Print and shaded views of the part. All mm, measured from the part's lowest x, y and z. A direction names the side the tool comes from. Round coordinates to 2 decimals unless told otherwise and drop trailing zeros. Write each loop counter-clockwise with the first axis right and the second up, starting at its lowest first coordinate (ties: lowest second). Pieces come first, ordered by that corner, then holes. Notation, with made-up numbers: M -5.5,-19 L 35.5,-19 A25 ccw 35.5,18 Z; hole C 45,-12 d5. An arc over 180 degrees is marked long. Write item = value, one per line. Start each with the question number.
Q1. Tool access for the marked faces 1, 2 and 3: list every direction of +Z, -Z, +X, -X, +Y, -Y with a clear straight run to the whole face (end or side of a thin tool).
Q2. Band-saw the part on D-D on y = 8.5. Write the cut outline in (x, z), plus the area to 3 significant figures.
Q3. Drop flat-ended pins along their axis: P1, Ø0.8, axis at y = 5, z = 4, coming from the -X side; P2, Ø8, axis at x = 9.5, y = 22.5, coming from the -Z side; P3, Ø3, axis at y = 6, z = 3.5, coming from the +X side; P4, Ø6, axis at y = 45, z = 8, coming from the -X side. Give the stop position or say it passes through.
Q4. Band-saw the part on B-B on y = 25.4. Write the cut outline in (x, z).
Q5. Pull direction X, two halves, no side cores. Call the marked faces 4, 5, 6 and 7: released by +X, released by -X, zero draft, split by the parting line, or undercut.
Q6. Band-saw the part on C-C on z = 16.5. Write the cut outline in (x, y), plus the area to 3 significant figures.
Q7. Band-saw the part on A-A on x = 38.1. Write the cut outline in (y, z).
Q8. Probe L1, parallel to X at y = 25.4, z = 9; L2, parallel to Y at x = 38.1, z = 14.25; L3, parallel to Z at x = 20, y = 42.5. List the from-to ranges inside material, lowest first.
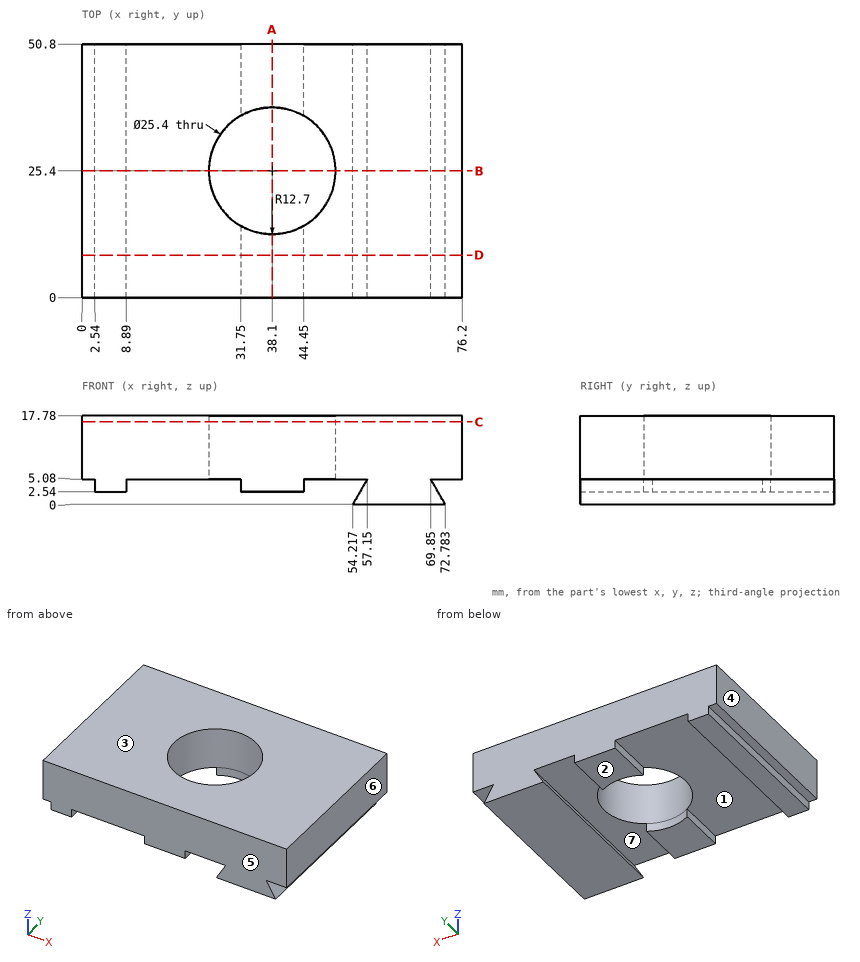
Conclusion:
q1.face_1 = -Z, +Y, -Y
q1.face_2 = -Z, -X, +Y, -Y
q1.face_3 = +Z, +X, -X, +Y, -Y
q2.outline = M 0,5.08 L 2.54,5.08 L 2.54,2.54 L 8.89,2.54 L 8.89,5.08 L 31.75,5.08 L 31.75,2.54 L 44.45,2.54 L 44.45,5.08 L 57.15,5.08 L 54.22,0 L 72.78,0 L 69.85,5.08 L 76.2,5.08 L 76.2,17.78 L 0,17.78 Z
q2.area = 1,100 mm^2
q3.P1 = 2.54
q3.P2 = 2.54
q3.P3 = 71.63
q3.P4 = 0
q4.outline = M 0,5.08 L 2.54,5.08 L 2.54,2.54 L 8.89,2.54 L 8.89,5.08 L 25.4,5.08 L 25.4,17.78 L 0,17.78 Z; M 50.8,5.08 L 57.15,5.08 L 54.22,0 L 72.78,0 L 69.85,5.08 L 76.2,5.08 L 76.2,17.78 L 50.8,17.78 Z
q5.face_4 = released by -X
q5.face_5 = zero draft
q5.face_6 = released by +X
q5.face_7 = undercut
q6.outline = M 0,0 L 76.2,0 L 76.2,50.8 L 0,50.8 Z; hole C 38.1,25.4 d25.4
q6.area = 3,360 mm^2
q7.outline = M 0,2.54 L 12.7,2.54 L 12.7,17.78 L 0,17.78 Z; M 38.1,2.54 L 50.8,2.54 L 50.8,17.78 L 38.1,17.78 Z
q8.L1 = 0 to 25.4, 50.8 to 76.2
q8.L2 = 0 to 12.7, 38.1 to 50.8
q8.L3 = 5.08 to 17.78
